from build123d import *

# Parameters (mm, degrees)
SKETCH1_W           = 160
SKETCH1_H           = 144
SKETCH1_R           = 2.5
BOSS_EXTRUDE1_DEPTH = 15.875
BOSS_EXTRUDE2_DEPTH = 15.875
BOSS_EXTRUDE3_DEPTH = 15.875
FILLET2_R           = 10
SKETCH4_R           = 2.5
CUT_EXTRUDE1_DEPTH  = 314.466131544
FILLET3_R           = 1
SKETCH5_R           = 2.5
CUT_EXTRUDE2_DEPTH  = 314.466131544
FILLET4_R           = 2
SKETCH6_R           = 11
CUT_EXTRUDE3_DEPTH  = 314.466131544
FILLET5_R           = 3


with BuildPart() as part:
    # Sketch1 → Boss-Extrude1 (new body)
    with BuildSketch(Plane.XY):
        Rectangle(SKETCH1_W, SKETCH1_H)
        with Locations((-58, -66)):
            Circle(SKETCH1_R, mode=Mode.SUBTRACT)
        with Locations((-22, -66)):
            Circle(SKETCH1_R, mode=Mode.SUBTRACT)
        with Locations((-58, -34)):
            Circle(SKETCH1_R, mode=Mode.SUBTRACT)
        with Locations((-22, -34)):
            Circle(SKETCH1_R, mode=Mode.SUBTRACT)
        with Locations(Location((58, -66, 0), (0, 0, 180))):
            Circle(SKETCH1_R, mode=Mode.SUBTRACT)
        with Locations(Location((22, -66, 0), (0, 0, 180))):
            Circle(SKETCH1_R, mode=Mode.SUBTRACT)
        with Locations(Location((22, -34, 0), (0, 0, 180))):
            Circle(SKETCH1_R, mode=Mode.SUBTRACT)
        with Locations(Location((58, -34, 0), (0, 0, 180))):
            Circle(SKETCH1_R, mode=Mode.SUBTRACT)
        with Locations(Location((-58, 66, 0), (0, 0, 180))):
            Circle(SKETCH1_R, mode=Mode.SUBTRACT)
        with Locations(Location((-22, 66, 0), (0, 0, 180))):
            Circle(SKETCH1_R, mode=Mode.SUBTRACT)
        with Locations((22, 66)):
            Circle(SKETCH1_R, mode=Mode.SUBTRACT)
        with Locations((58, 66)):
            Circle(SKETCH1_R, mode=Mode.SUBTRACT)
        with Locations((58, 34)):
            Circle(SKETCH1_R, mode=Mode.SUBTRACT)
        with Locations((22, 34)):
            Circle(SKETCH1_R, mode=Mode.SUBTRACT)
        with Locations(Location((-22, 34, 0), (0, 0, 180))):
            Circle(SKETCH1_R, mode=Mode.SUBTRACT)
        with Locations(Location((-58, 34, 0), (0, 0, 180))):
            Circle(SKETCH1_R, mode=Mode.SUBTRACT)
    extrude(amount=BOSS_EXTRUDE1_DEPTH)

    # Sketch2 → Boss-Extrude2 (add, through all)
    with BuildSketch(Plane.XY.offset(15.875)):
        Polygon((55, 272), (155, 272), (155, 152), (80, 152), (80, 72), (-80, 72), (-80, 122), align=None)
    extrude(amount=-BOSS_EXTRUDE2_DEPTH)

    # Sketch3 → Boss-Extrude3 (add, through all)
    with BuildSketch(Plane.XY.offset(15.875)):
        Polygon((155, 152), (80, 65.589776693), (80, 152), align=None)
    extrude(amount=-BOSS_EXTRUDE3_DEPTH)

    # Fillet2
    fillet2_edges = [part.edges().sort_by_distance(p)[0] for p in [
        (80, 65.589776693, 7.9375),
        (-80, 122, 7.9375),
        (55, 272, 7.9375),
    ]]
    fillet(fillet2_edges, radius=FILLET2_R)

    # Sketch4 → Cut-Extrude1 (cut, through all)
    with BuildSketch(Plane.XY.offset(15.875)):
        with Locations((-32, 20)):
            Circle(SKETCH4_R)
        with Locations(Location((-8, 20, 0), (0, 0, 180))):
            Circle(SKETCH4_R)
        with Locations((-8, -20)):
            Circle(SKETCH4_R)
        with Locations(Location((-32, -20, 0), (0, 0, 180))):
            Circle(SKETCH4_R)
    extrude(amount=-CUT_EXTRUDE1_DEPTH, mode=Mode.SUBTRACT)

    # Fillet3
    fillet3_edges = [part.edges().sort_by_distance(p)[0] for p in [
        (155, 272, 7.9375),
    ]]
    fillet(fillet3_edges, radius=FILLET3_R)

    # Sketch5 → Cut-Extrude2 (cut, through all)
    with BuildSketch(Plane.XY.offset(15.875)):
        with Locations((145, 262)):
            Circle(SKETCH5_R)
        with Locations((145, 242)):
            Circle(SKETCH5_R)
        with Locations((145, 222)):
            Circle(SKETCH5_R)
        with Locations((145, 202)):
            Circle(SKETCH5_R)
        with Locations((145, 182)):
            Circle(SKETCH5_R)
        with Locations((145, 162)):
            Circle(SKETCH5_R)
        with Locations((125, 162)):
            Circle(SKETCH5_R)
        with Locations((125, 262)):
            Circle(SKETCH5_R)
    extrude(amount=-CUT_EXTRUDE2_DEPTH, mode=Mode.SUBTRACT)

    # Fillet4
    fillet4_edges = [part.edges().sort_by_distance(p)[0] for p in [
        (155, 152, 7.9375),
    ]]
    fillet(fillet4_edges, radius=FILLET4_R)

    # Sketch6 → Cut-Extrude3 (cut, through all)
    with BuildSketch(Plane.XY.offset(15.875)):
        with Locations((105, 212)):
            Circle(SKETCH6_R)
    extrude(amount=-CUT_EXTRUDE3_DEPTH, mode=Mode.SUBTRACT)

    # Fillet5
    fillet5_edges = [part.edges().sort_by_distance(p)[0] for p in [
        (80, -72, 7.9375),
        (-80, -72, 7.9375),
    ]]
    fillet(fillet5_edges, radius=FILLET5_R)


solid = part.part
CAD build for the part. Positions are in the model's coordinates, mm. A direction names the side the tool comes from. Give positions to 0.01 mm unless a question says otherwise; leave off trailing zeros. Order: outer loops, then holes, each group sorted by start corner. A loop starts at its lowest first (then second) coordinate and runs counter-clockwise, first axis right, second up. Notation, with made-up numbers: (67, 5) - (104, 5) arc R34 cw to (104, 38) - close; hole circle Ø1 at (18.5, 49). An arc over 180 degrees is marked (long way). Write each question's results on one line, items separated by ' | '.
1. 3-axis set-ups, long thin cutter, end or side, ignore diameter. For faces 1 (the face through (-79.32, 121.79, 7.83)), 2 (the face through (80, -3, 8)): which of +Z, -Z, +X, -X, +Y, -Y reach the whole face in a straight line?
Calculated:
face 1: +Z, -Z, -X, +Y | face 2: +Z, -Z, +X, -Y
2. Pull direction X, two halves, no side cores. Call faces 3 (the face through (103.568, 222.906, 8.049)), 4 (the face through (-80, 23, 8)), 5 (the face through (39, 102, 0)): released by +X, released by -X, zero draft, split by the parting line, or undercut.
Calculated:
face 3: undercut | face 4: released by -X | face 5: zero draft
3. Saw through at A-A on z = 3.75. Count the separate pieces of the cut face and the enclosed holes in it, and give its area (3 significant figures).
Calculated:
separate pieces: 1 | enclosed holes: 29 | area: 56,200 mm2
4. Pin check, flat tips, straight feed: pin 1 (1.5 mm diameter, centred on x = 15.5, z = 3, fed in from +Y); pin 2 (5 mm diameter, centred on x = 87, y = 69, fed in from +Z); pin 3 (5 mm diameter, centred on y = 131, z = 11.5, fed in from -X); pin 4 (2 mm diameter, centred on y = -13.5, z = 2, fed in from +X). Stop position of each tip, or through.
Calculated:
pin 1: stops at y = 228.94 | pin 2: passes through | pin 3: stops at x = -74.15 | pin 4: stops at x = 80
5. Saw through at C-C on x = -49.5. List the corners of the cut face in (y, z) (3 decimals).
Calculated:
outline: (-72, 0) - (155.889, 0) - (155.889, 15.875) - (-72, 15.875) - close
6. Saw through at B-B on y = 28. List the corners of the cut face in (x, z) (3 decimals), and give its area (3 significant figures).
Calculated:
outline: (-80, 0) - (80, 0) - (80, 15.875) - (-80, 15.875) - close | area: 2,540 mm2
7. Probe L1, parallel to X at y = 262, z = 7; L2, parallel to X at y = 202, z = 9; L3, parallel to Y at x = -34, z = 14.75. List the from-to ranges inside material, lowest first. Write a range as from..to.
Calculated:
L1: x = 46..122.5, 127.5..142.5, 147.5..155 | L2: x = -8..100.42, 109.58..142.5, 147.5..155 | L3: y = -72..-21.5, -18.5..18.5, 21.5..173.11
